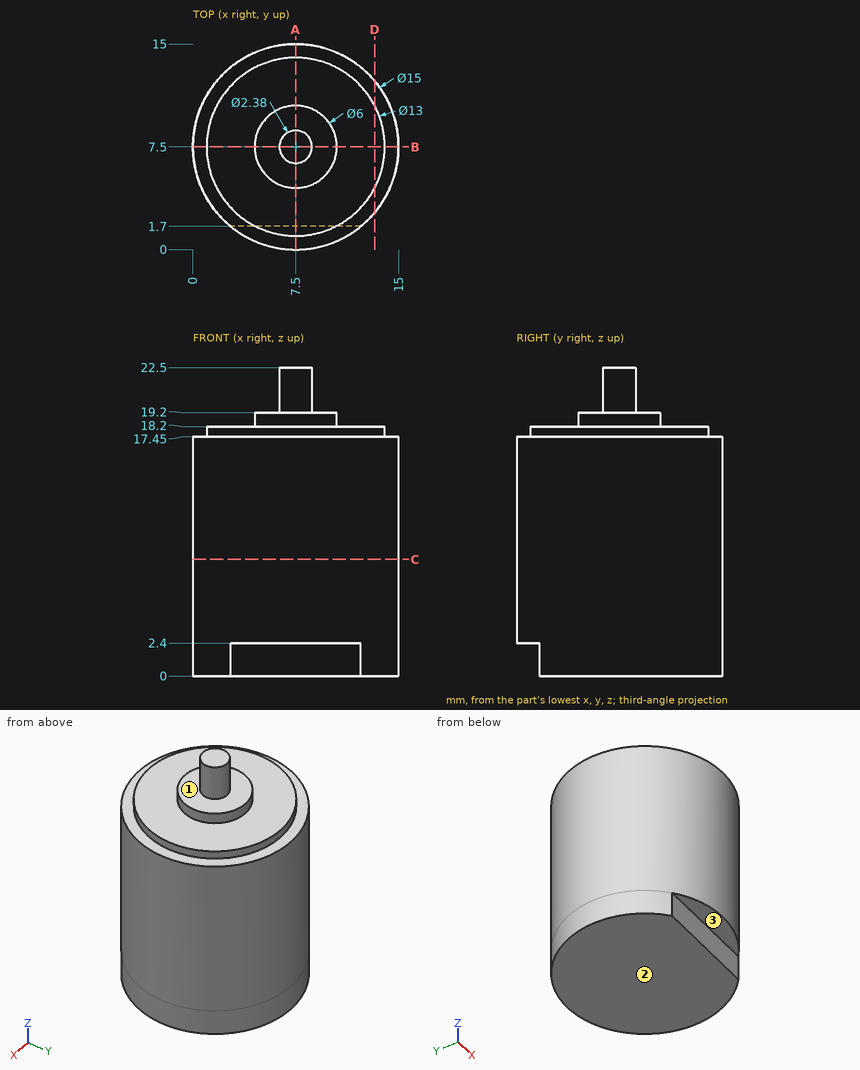
The drawing under review shows one solid part. Ordinate dimensions are in mm from its lowest x, y, z. A direction names the side the tool comes from. Coordinates: 2 decimals unless noted, no trailing zeros. Write each loop counter-clockwise with the first axis right and the second up, starting at its lowest first coordinate (ties: lowest second). Pieces come first, ordered by that corner, then holes. Notation, with made-up numbers: (57, -25.75) - (67, -25.75) arc R33 ccw to (67, 10.25) - close; hole circle Ø6 at (81, -25). An arc over 180 degrees is marked (long way). Use one line per item in the form item = value.
Q1. Machinability: for the marked faces 1, 2 and 3, which of the approach directions +Z, -Z, +X, -X, +Y, -Y give a long, thin tool a straight path to every point of the face, cutting with its end or side? Answer none if there is none.
Taken from the geometry:
face_1 = +Z
face_2 = -Z, +X, -X, +Y, -Y
face_3 = -Z, +X, -X, -Y
Q2. Consider section A-A (x = 7.5). Write out the cut boundary in (y, z), plus the area to 3 significant figures.
Taken from the geometry:
outline = (0, 2.4) - (1.7, 2.4) - (1.7, 0) - (15, 0) - (15, 17.45) - (14, 17.45) - (14, 18.2) - (10.5, 18.2) - (10.5, 19.2) - (8.69, 19.2) - (8.69, 22.5) - (6.31, 22.5) - (6.31, 19.2) - (4.5, 19.2) - (4.5, 18.2) - (1, 18.2) - (1, 17.45) - (0, 17.45) - close
area = 281 mm^2
Q3. Insertion check: pin 1 Ø1.9 at (x, z) = (8.5, 1) entering from -Y; pin 2 Ø0.5 at (x, y) = (7, 1) entering from -Z; pin 3 Ø5 at (x, z) = (4, 13) entering from +Y. Each pin has a flat end and moves straight along its axis. Give the tip position at first contact, or say it passes through.
Taken from the geometry:
pin_1 = 1.7
pin_2 = 2.4
pin_3 = 14.93
Q4. Consider section D-D (x = 13.25). Write out the cut boundary in (y, z), plus the area to 3 significant figures.
Taken from the geometry:
outline = (2.68, 0) - (12.32, 0) - (12.32, 17.45) - (10.53, 17.45) - (10.53, 18.2) - (4.47, 18.2) - (4.47, 17.45) - (2.68, 17.45) - close
area = 173 mm^2
Q5. Consider section B-B (y = 7.5). Write out the cut boundary in (x, z), plus the area to 3 significant figures.
Taken from the geometry:
outline = (0, 0) - (15, 0) - (15, 17.45) - (14, 17.45) - (14, 18.2) - (10.5, 18.2) - (10.5, 19.2) - (8.69, 19.2) - (8.69, 22.5) - (6.31, 22.5) - (6.31, 19.2) - (4.5, 19.2) - (4.5, 18.2) - (1, 18.2) - (1, 17.45) - (0, 17.45) - close
area = 285 mm^2
Q6. For probe 1 along Z at (x, y) = (12, 6.75); probe 2 along Y at (x, z) = (7.75, 3.5); probe 3 along Z at (x, y) = (8, 9.5), list the stretches that pass through material, from the lowest coordinate up.
Taken from the geometry:
probe_1 = 0 to 18.2
probe_2 = 0 to 15
probe_3 = 0 to 19.2
Q7. Consider section C-C (z = 8.5). Write out the cut boundary in (x, y), plus the area to 3 significant figures.
Taken from the geometry:
outline = circle Ø15 at (7.5, 7.5)
area = 177 mm^2
